Check sheet for the modelled part. Datum: model origin and axes. Units: mm. Round coordinates to 2 decimals unless told otherwise and drop trailing zeros. Loops run counter-clockwise (first coordinate to the right, second up) from the corner with the lowest first, then second, coordinate; pieces in that order, holes last. Notation, with made-up numbers: M 58.5,22 L 88.5,22 A16 ccw 88.5,33 Z; hole C 23,8.25 d1. An arc over 180 degrees is marked long. Write item = value, one per line. Start each with the question number.
(1) Cross-section at B-B on x = 68. Record the boundary of the cut face in (y, z).
(2) Cross-section at D-D on z = 0.95. State how many separate pieces and enclosed holes the cut face has, plus the area to 3 significant figures.
(3) Go/stop test with flat-tipped pins: P1, Ø7, axis at x = 111.46, y = -43.81, coming from the -Z side; P2, Ø1.5, axis at x = 69, z = 2, coming from the +Y side. Record where each tip stops, or that it passes through.
(4) Scan lines: L1, parallel to Y at x = 128.5, z = 2.15; L2, parallel to X at y = -37.5, z = 0.4; L3, parallel to Y at x = 33, z = 1.5. Record each from-to range of solid material in increasing order. Write a range as from..to.
(5) Cross-section at A-A on x = 128.5. Record the boundary of the cut face in (y, z).
(6) Cross-section at C-C on x = 89. Record the boundary of the cut face in (y, z).
from build123d import *

# Parameters (mm, degrees)
F0_W     = 145
F0_H     = 75
F0_R     = 4
F0_R_2   = 5
F0_W_2   = 20
F0_H_2   = 20
F0_W_3   = 12
F1_DEPTH = 3
F2_DEPTH = 1


with BuildPart() as f1:
    # F0 (on Top) → F1 (new body)
    with BuildSketch(Plane.XY):
        with Locations((72.5, -37.5)):
            Rectangle(F0_W, F0_H)
        with Locations((17.5, -63.5)):
            Circle(F0_R, mode=Mode.SUBTRACT)
        with Locations((33, -63.5)):
            Circle(F0_R, mode=Mode.SUBTRACT)
        with Locations((47, -63.5)):
            Circle(F0_R, mode=Mode.SUBTRACT)
        with Locations((61, -63.5)):
            Circle(F0_R, mode=Mode.SUBTRACT)
        with Locations((17.5, -44.955306)):
            Circle(F0_R_2, mode=Mode.SUBTRACT)
        with Locations((40.5, -42.5)):
            Rectangle(F0_W_2, F0_H_2, mode=Mode.SUBTRACT)
        with Locations((65.5, -42.5)):
            Rectangle(F0_W_2, F0_H_2, mode=Mode.SUBTRACT)
        with Locations((75, -63.5)):
            Circle(F0_R, mode=Mode.SUBTRACT)
        with Locations((89, -63.5)):
            Circle(F0_R, mode=Mode.SUBTRACT)
        with Locations((103, -63.5)):
            Circle(F0_R, mode=Mode.SUBTRACT)
        with Locations((117, -63.5)):
            Circle(F0_R, mode=Mode.SUBTRACT)
        with Locations((128.5, -63.5)):
            Circle(F0_R, mode=Mode.SUBTRACT)
        with Locations((90.5, -42.5)):
            Rectangle(F0_W_2, F0_H_2, mode=Mode.SUBTRACT)
        with Locations((111.459419, -43.807857)):
            Circle(F0_R, mode=Mode.SUBTRACT)
        with Locations((128.5, -43.807857)):
            Circle(F0_R_2, mode=Mode.SUBTRACT)
        with Locations((17.5, -19.316503)):
            Circle(F0_R_2, mode=Mode.SUBTRACT)
        with Locations((40.5, -17.5)):
            Rectangle(F0_W_2, F0_H_2, mode=Mode.SUBTRACT)
        with Locations((65.5, -17.5)):
            Rectangle(F0_W_2, F0_H_2, mode=Mode.SUBTRACT)
        with Locations((128.5, -19.316503)):
            Circle(F0_R, mode=Mode.SUBTRACT)
        with Locations((90.5, -17.5)):
            Rectangle(F0_W_2, F0_H_2, mode=Mode.SUBTRACT)
        with Locations((111.5, -17.5)):
            Rectangle(F0_W_3, F0_H_2, mode=Mode.SUBTRACT)
    extrude(amount=F1_DEPTH)


with BuildPart() as f2:
    # F0 (on Top) → F2 (new body)
    with BuildSketch(Plane.XY):
        with Locations((72.5, -37.5)):
            Rectangle(F0_W, F0_H)
        with Locations((17.5, -63.5)):
            Circle(F0_R, mode=Mode.SUBTRACT)
        with Locations((33, -63.5)):
            Circle(F0_R, mode=Mode.SUBTRACT)
        with Locations((47, -63.5)):
            Circle(F0_R, mode=Mode.SUBTRACT)
        with Locations((61, -63.5)):
            Circle(F0_R, mode=Mode.SUBTRACT)
        with Locations((17.5, -44.955306)):
            Circle(F0_R_2, mode=Mode.SUBTRACT)
        with Locations((40.5, -42.5)):
            Rectangle(F0_W_2, F0_H_2, mode=Mode.SUBTRACT)
        with Locations((65.5, -42.5)):
            Rectangle(F0_W_2, F0_H_2, mode=Mode.SUBTRACT)
        with Locations((75, -63.5)):
            Circle(F0_R, mode=Mode.SUBTRACT)
        with Locations((89, -63.5)):
            Circle(F0_R, mode=Mode.SUBTRACT)
        with Locations((103, -63.5)):
            Circle(F0_R, mode=Mode.SUBTRACT)
        with Locations((117, -63.5)):
            Circle(F0_R, mode=Mode.SUBTRACT)
        with Locations((128.5, -63.5)):
            Circle(F0_R, mode=Mode.SUBTRACT)
        with Locations((90.5, -42.5)):
            Rectangle(F0_W_2, F0_H_2, mode=Mode.SUBTRACT)
        with Locations((111.459419, -43.807857)):
            Circle(F0_R, mode=Mode.SUBTRACT)
        with Locations((128.5, -43.807857)):
            Circle(F0_R_2, mode=Mode.SUBTRACT)
        with Locations((17.5, -19.316503)):
            Circle(F0_R_2, mode=Mode.SUBTRACT)
        with Locations((40.5, -17.5)):
            Rectangle(F0_W_2, F0_H_2, mode=Mode.SUBTRACT)
        with Locations((65.5, -17.5)):
            Rectangle(F0_W_2, F0_H_2, mode=Mode.SUBTRACT)
        with Locations((128.5, -19.316503)):
            Circle(F0_R, mode=Mode.SUBTRACT)
        with Locations((90.5, -17.5)):
            Rectangle(F0_W_2, F0_H_2, mode=Mode.SUBTRACT)
        with Locations((111.5, -17.5)):
            Rectangle(F0_W_3, F0_H_2, mode=Mode.SUBTRACT)
    extrude(amount=-F2_DEPTH)


solid = f1.part
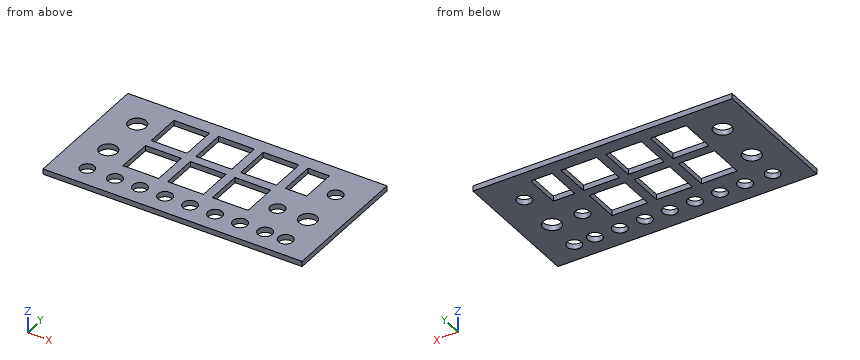
Result:
q1.outline = M -75,0 L -52.5,0 L -52.5,3 L -75,3 Z; M -32.5,0 L -27.5,0 L -27.5,3 L -32.5,3 Z; M -7.5,0 L 0,0 L 0,3 L -7.5,3 Z
q2.separate_pieces = 1
q2.enclosed_holes = 21
q2.area = 7,450 mm^2
q3.P1 = through
q3.P2 = 0
q4.L1 = -75..-67.5, -59.5..-48.81, -38.81..-23.32, -15.32..0
q4.L2 = 0..30.5, 50.5..55.5, 75.5..80.5, 100.5..145
q4.L3 = -75..-67.5, -59.5..-52.5, -32.5..-27.5, -7.5..0
q5.outline = M -75,0 L -67.5,0 L -67.5,3 L -75,3 Z; M -59.5,0 L -48.81,0 L -48.81,3 L -59.5,3 Z; M -38.81,0 L -23.32,0 L -23.32,3 L -38.81,3 Z; M -15.32,0 L 0,0 L 0,3 L -15.32,3 Z
q6.outline = M -75,0 L -67.5,0 L -67.5,3 L -75,3 Z; M -59.5,0 L -52.5,0 L -52.5,3 L -59.5,3 Z; M -32.5,0 L -27.5,0 L -27.5,3 L -32.5,3 Z; M -7.5,0 L 0,0 L 0,3 L -7.5,3 Z
